Read the model definition and answer for the solid it produces. Units are mm, in the model's axes. Face numbers are marked on the shaded views. A direction names the side the tool comes from. Coordinates: 2 decimals unless noted, no trailing zeros. Loops run counter-clockwise (first coordinate to the right, second up) from the corner with the lowest first, then second, coordinate; pieces in that order, holes last. Notation, with made-up numbers: M 7.25,-37.5 L 32.25,-37.5 A24 ccw 32.25,-8.5 Z; hole C 50,24.25 d7. An arc over 180 degrees is marked long. Put each result on its own line as item: value.
from build123d import *

# Parameters (mm, degrees)
SKETCH1_W           = 20
SKETCH1_H           = 49.25
BOSS_EXTRUDE1_DEPTH = 2.5
FILLET3_R           = 2.5
CUT_EXTRUDE1_DEPTH  = 51.317119353
SKETCH14_R          = 2
BOSS_EXTRUDE2_DEPTH = 5.5


with BuildPart() as part:
    # Sketch1 → Boss-Extrude1 (new, symmetric)
    with BuildSketch(Plane.XY):
        with Locations((0, 24.625)):
            Rectangle(SKETCH1_W, SKETCH1_H)
    extrude(amount=BOSS_EXTRUDE1_DEPTH, both=True)

    # Fillet3
    fillet3_edges = [part.edges().sort_by_distance(p)[0] for p in [
        (10, 24.625, 2.5),
        (10, 24.625, -2.5),
    ]]
    fillet(fillet3_edges, radius=FILLET3_R - 0.0001)  # a hair under: the kernel refuses the full size

    # Sketch11 → Cut-Extrude1 (cut, through all)
    with BuildSketch(Plane(origin=(0, 49.25, 0), x_dir=(1, 0, 0), z_dir=(0, 1, 0))):
        Polygon((-10, 1), (7.5, 2.5), (-10, 2.5), align=None)
        Polygon((7.5, -2.5), (-10, -1), (-10, -2.5), align=None)
    extrude(amount=-CUT_EXTRUDE1_DEPTH, mode=Mode.SUBTRACT)

    # Sketch14 → Boss-Extrude2 (add, symmetric)
    with BuildSketch(Plane.XY):
        with Locations((0, 39.25)):
            Circle(SKETCH14_R)
    extrude(amount=BOSS_EXTRUDE2_DEPTH, both=True)


solid = part.part
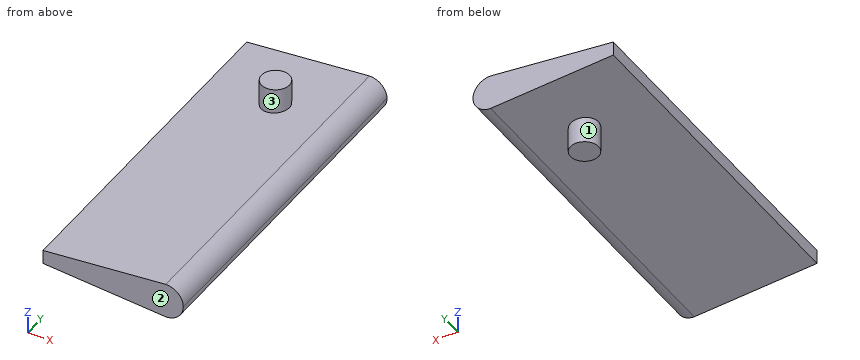
1) Find section B-B, the plane x = -0.75. Write down the section's boundary in (y, z).
Answer list:
outline: M 0,-1.79 L 37.4,-1.79 L 37.4,-5.5 L 41.1,-5.5 L 41.1,-1.79 L 49.25,-1.79 L 49.25,1.79 L 41.1,1.79 L 41.1,5.5 L 37.4,5.5 L 37.4,1.79 L 0,1.79 Z
2) Straight lines are drawn through the part: line 1 (Z direction, x = -2, y = 19); line 2 (Z direction, x = -0.5, y = 5.5); line 3 (X direction, y = 36.5, z = -0.75). For each, find the intervals that lie inside material, in ascending order. Write a range as [from, to].
Answer list:
line 1: z = [-1.69, 1.69]
line 2: z = [-1.81, 1.81]
line 3: x = [-10, 9.88]
3) Given pin 1 Ø4 at (x, z) = (2.5, 1.5) entering from -Y; pin 2 Ø4 at (x, y) = (-4.5, 11.5) entering from +Z; pin 3 Ø3 at (x, y) = (7, 33.5) entering from -Z; pin 4 Ø12 at (x, y) = (-4, 12.5) entering from -Z, each flat-ended and moving along its own axis, determine where each tip first touches the part or whether it passes through.
Answer list:
pin 1: stops at y = 0
pin 2: stops at z = 1.64
pin 3: stops at z = -2.5
pin 4: stops at z = -2.03
4) Find section C-C, the plane z = 3.5. Write down the section's boundary in (x, y).
Answer list:
outline: C 0,39.25 d4
5) Which of the six approach directions +Z, -Z, +X, -X, +Y, -Y give full straight-line access (tool end or side, diameter ignored) to the marked faces 1, 2 and 3?
Answer list:
face 1: -Z
face 2: +Z, -Z, +X, -X, -Y
face 3: +Z
